from build123d import *

# Parameters (mm, degrees)
BOSS_EXTRUDE1_DEPTH = 2
SKETCH3_R           = 1.05
CUT_EXTRUDE1_DEPTH  = 2
SKETCH4_W           = 5
SKETCH4_H           = 9
BOSS_EXTRUDE2_DEPTH = 9
SKETCH5_W           = 2.6
SKETCH5_H           = 5
BOSS_EXTRUDE3_DEPTH = 4


with BuildPart() as part:
    # Sketch2 → Boss-Extrude1 (new body)
    with BuildSketch(Plane(origin=(0, 0, 0), x_dir=(1, 0, 0), z_dir=(0, 1, 0))):
        Polygon((0, 0), (5.5, 0), (5.5, 89), (4.5, 89), (0, 74), align=None)
    extrude(amount=BOSS_EXTRUDE1_DEPTH)

    # Mirror1: part across plane


with BuildPart() as part_1:
    add(part.part)
    add(part.part.mirror(Plane(origin=(5.5, 2, 0), x_dir=(0, 0, 1), z_dir=(-1, 0, 0))))

    # Sketch3 → Cut-Extrude1 (cut)
    with BuildSketch(Plane(origin=(0, 2, 0), x_dir=(1, 0, 0), z_dir=(0, 1, 0))):
        with Locations((5.5, 9)):
            Circle(SKETCH3_R)
        with Locations((5.5, 24.5)):
            Circle(SKETCH3_R)
        with Locations((5.5, 49)):
            Circle(SKETCH3_R)
        with Locations((5.5, 63.5)):
            Circle(SKETCH3_R)
    extrude(amount=-CUT_EXTRUDE1_DEPTH, mode=Mode.SUBTRACT)

    # Sketch4 → Boss-Extrude2 (add)
    with BuildSketch(Plane(origin=(0, 2, 0), x_dir=(1, 0, 0), z_dir=(0, 1, 0))):
        with Locations((5.5, 37.5)):
            Rectangle(SKETCH4_W, SKETCH4_H)
    extrude(amount=BOSS_EXTRUDE2_DEPTH)

    # Sketch5 → Boss-Extrude3 (add)
    with BuildSketch(Plane(origin=(0, 11, 0), x_dir=(1, 0, 0), z_dir=(0, 1, 0))):
        with Locations((5.5, 37.5)):
            Rectangle(SKETCH5_W, SKETCH5_H)
    extrude(amount=BOSS_EXTRUDE3_DEPTH)


solid = part_1.part
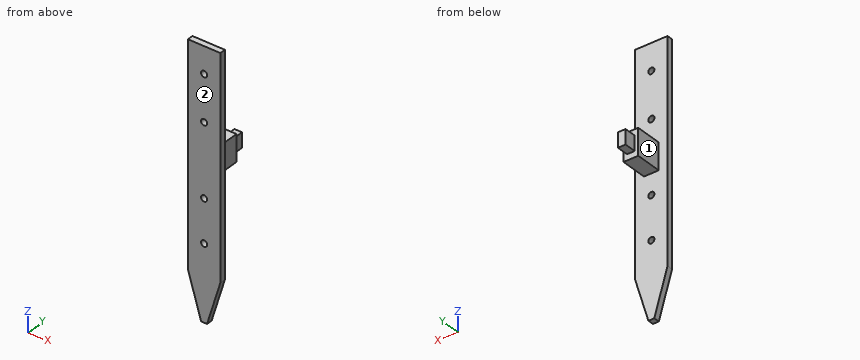
Can you work these out from the model? Positions are in its coordinate system, mm. Face numbers are marked on the shaded views. A direction names the side the tool comes from. Give positions to 0.01 mm unless a question says otherwise; leave off trailing zeros. Write each loop counter-clockwise with the first axis right and the second up, starting at its lowest first coordinate (ties: lowest second). Pieces come first, ordered by that corner, then holes. Notation, with made-up numbers: (-13, 67) -> (4, 67) arc R8 cw to (4, 80) -> close; hole circle Ø7 at (87, 39). An arc over 180 degrees is marked (long way). Answer as a JSON object with one key per item and string values. Group by question number.
Item 1: For the marked faces 1 and 2, which set-ups out of +Z, -Z, +X, -X, +Y, -Y let a thin tool reach every point of the face, with its end or its side?
Item 2: Please list where these lines run through material, in increasing order: line 1 (Z direction, x = 5.5, y = 1.5); line 2 (Z direction, x = 5, y = 1.25); line 3 (X direction, y = 1.6, z = -24.5). Write a range as [from, to].
Item 3: I'm going to push flat-ended pins straight in: P1, Ø4, axis at y = 2.5, z = -17, coming from the -X side; P2, Ø1.3, axis at x = 6, y = 13.5, coming from the -Z side; P3, Ø4.5, axis at y = 6.5, z = -36, coming from the -X side; P4, Ø1.5, axis at x = 6, y = 6, coming from the -Z side. Where does each tip first touch, or does it pass through?
Item 4: Suppose I cut it at C-C (y = 1). Please give me the cut outline in (x, z).
Item 5: Suppose I cut it at D-D (x = 9.5). Please give me the cut outline in (y, z), plus the area to 3 significant figures.
Item 6: Suppose I cut it at A-A (z = -9). Please give me the cut outline in (x, y), plus the area to 3 significant figures.
Item 7: Suppose I cut it at B-B (x = 5.5). Please give me the cut outline in (y, z).
Findings:
{
 "1": {"face 1": "+Z, -Z, -X, +Y", "face 2": "+Z, -Z, +X, -X, -Y"},
 "2": {"line 1": "z = [-89, -64.55], [-62.45, -50.05], [-47.95, -25.55], [-23.45, -10.05], [-7.95, 0]", "line 2": "z = [-89, -64.42], [-62.58, -49.92], [-48.08, -25.42], [-23.58, -9.92], [-8.08, 0]", "line 3": "x = [0, 4.45], [6.55, 11]"},
 "3": {"P1": "stops at x = 0", "P2": "stops at z = -40", "P3": "stops at x = 3", "P4": "stops at z = -42"},
 "4": {"outline": "(0, -74) -> (4.5, -89) -> (6.5, -89) -> (11, -74) -> (11, 0) -> (0, 0) -> close; hole circle Ø2.1 at (5.5, -63.5); hole circle Ø2.1 at (5.5, -49); hole circle Ø2.1 at (5.5, -24.5); hole circle Ø2.1 at (5.5, -9)"},
 "5": {"outline": "(0, -79) -> (2, -79) -> (2, 0) -> (0, 0) -> close", "area": "158 mm²"},
 "6": {"outline": "(0, 0) -> (4.45, 0) -> (4.45, 2) -> (0, 2) -> close; (6.55, 0) -> (11, 0) -> (11, 2) -> (6.55, 2) -> close", "area": "17.8 mm²"},
 "7": {"outline": "(0, -89) -> (2, -89) -> (2, -64.55) -> (0, -64.55) -> close; (0, -62.45) -> (2, -62.45) -> (2, -50.05) -> (0, -50.05) -> close; (0, -47.95) -> (2, -47.95) -> (2, -42) -> (11, -42) -> (11, -40) -> (15, -40) -> (15, -35) -> (11, -35) -> (11, -33) -> (2, -33) -> (2, -25.55) -> (0, -25.55) -> close; (0, -23.45) -> (2, -23.45) -> (2, -10.05) -> (0, -10.05) -> close; (0, -7.95) -> (2, -7.95) -> (2, 0) -> (0, 0) -> close"}
}
